Geometry check sheet. Reference: the model listing, model coordinates, mm. Face numbers are marked on the shaded views. A direction names the side the tool comes from. Round coordinates to 2 decimals unless told otherwise and drop trailing zeros. Order: outer loops, then holes, each group sorted by start corner. A loop starts at its lowest first (then second) coordinate and runs counter-clockwise, first axis right, second up. Notation, with made-up numbers: (84.25, -30.5) -> (103.25, -30.5) arc R22 cw to (103.25, -20.5) -> close; hole circle Ø5 at (72.5, 72.25). An arc over 180 degrees is marked (long way). Use a Markdown table: item, result. Add a question column.
Item 1: Material ranges on probe 1 along Z at (x, y) = (0, 3.75); probe 2 along X at (y, z) = (2.25, 0.75); probe 3 along X at (y, z) = (0.5, 1.75), recorded low to high. Write a range as [from, to].
Item 2: Sectioned sample at B-B, the plane z = 0. Record the cut outline in (x, y).
Item 3: Sectioned sample at A-A, the plane x = -11. Record the cut outline in (y, z), and give its area (3 significant figures).
Item 4: Gauge pin test, flat ends, axial feed: pin 1 Ø3 at (y, z) = (8, -1.5) entering from +X; pin 2 Ø0.8 at (x, z) = (0.5, -0.5) entering from +Y. Record the tip position at first contact, or that the pin passes through.
Item 5: Sectioned sample at D-D, the plane y = 4.75. Record the cut outline in (x, z), and give its area (3 significant figures).
Item 6: Sectioned sample at C-C, the plane x = 0. Record the cut outline in (y, z).
Item 7: Set-up check for the marked faces 1 and 2: record each of +Z, -Z, +X, -X, +Y, -Y from which the full face is reachable in a straight line by a thin tool's end or side.
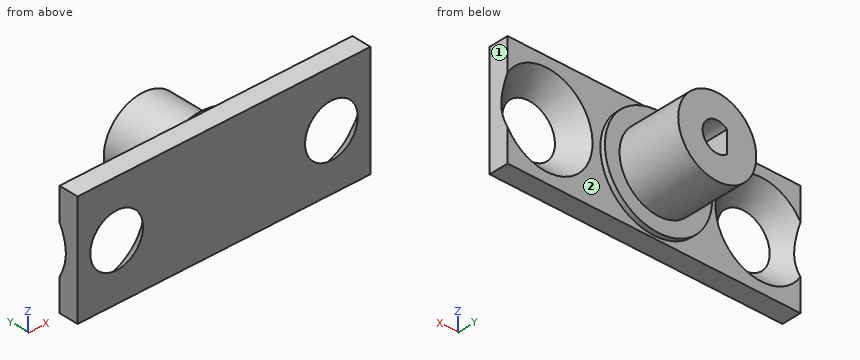
from build123d import *

# Parameters (mm, degrees)
SKETCH1_W                                    = 30
SKETCH1_H                                    = 11.5
BOSS_EXTRUDE1_DEPTH                          = 2
SKETCH2_R                                    = 5.5
BOSS_EXTRUDE2_DEPTH                          = 0.5
SKETCH3_R                                    = 4
BOSS_EXTRUDE3_DEPTH                          = 6.5
CUT_EXTRUDE1_DEPTH                           = 7
CSK_FOR_M4_COUNTERSUNK_FLAT_HEAD_SCR_2_COUNT = 2
CSK_FOR_M4_COUNTERSUNK_FLAT_HEAD_SCR_2_PITCH = 22


with BuildPart() as part:
    # Sketch1 → Boss-Extrude1 (new body)
    with BuildSketch(Plane(origin=(0, 0, 0), x_dir=(1, 0, 0), z_dir=(0, 1, 0))):
        Rectangle(SKETCH1_W, SKETCH1_H)
    extrude(amount=BOSS_EXTRUDE1_DEPTH)

    # Sketch2 → Boss-Extrude2 (add)
    with BuildSketch(Plane(origin=(0, 2, 0), x_dir=(1, 0, 0), z_dir=(0, 1, 0))):
        Circle(SKETCH2_R)
    extrude(amount=BOSS_EXTRUDE2_DEPTH)

    # Sketch3 → Boss-Extrude3 (add)
    with BuildSketch(Plane(origin=(0, 2.5, 0), x_dir=(1, 0, 0), z_dir=(0, 1, 0))):
        Circle(SKETCH3_R)
    extrude(amount=BOSS_EXTRUDE3_DEPTH)

    # Sketch4 → Cut-Extrude1 (cut)
    with BuildSketch(Plane(origin=(0, 9, 0), x_dir=(1, 0, 0), z_dir=(0, 1, 0))):
        with BuildLine():
            Line((-1, 1.118033989), (-1, -1.118033989))
            ThreePointArc((-1, -1.118033989), (1.5, 0), (-1, 1.118033989))
        make_face()
    extrude(amount=-CUT_EXTRUDE1_DEPTH, mode=Mode.SUBTRACT)

    # Sketch6 → CSK for M4 Countersunk Flat Head Screw1 (revolve, cut)
    with BuildSketch(Plane(origin=(11, 2, 0), x_dir=(0, 0, 1), z_dir=(1, 0, 0))):
        Polygon((0, 0), (0, 3.351936393), (2.25, 2), (2.25, 2.45), (4.7, 0), align=None)
    csk_for_m4_countersunk_flat_head_screw1 = revolve(axis=Axis((11, 8.35, 0), (0, -1, 0)), mode=Mode.SUBTRACT)

    # CSK for M4 Countersunk Flat Head Scr 2: CSK for M4 Countersunk Flat Head Screw1 ×2
    with Locations(*[(-i * CSK_FOR_M4_COUNTERSUNK_FLAT_HEAD_SCR_2_PITCH, 0, 0) for i in range(1, CSK_FOR_M4_COUNTERSUNK_FLAT_HEAD_SCR_2_COUNT)]):
        add(csk_for_m4_countersunk_flat_head_screw1, mode=Mode.SUBTRACT)


solid = part.part
Found:
| question | item | result |
|---|---|---|
| 1 | probe 1 | z = [-4, -1.5], [1.5, 4] |
| 1 | probe 2 | x = [-5.45, -1], [1.3, 5.45] |
| 1 | probe 3 | x = [-15, -13.68], [-8.32, 8.32], [13.68, 15] |
| 2 | outline | (-15, 0) -> (-13.7, 0) -> (-15, 1.3) -> close; (-8.3, 0) -> (8.3, 0) -> (6.3, 2) -> (5.5, 2) -> (5.5, 2.5) -> (4, 2.5) -> (4, 9) -> (1.5, 9) -> (1.5, 2) -> (-1, 2) -> (-1, 9) -> (-4, 9) -> (-4, 2.5) -> (-5.5, 2.5) -> (-5.5, 2) -> (-6.3, 2) -> close; (13.7, 0) -> (15, 0) -> (15, 1.3) -> close |
| 3 | outline | (0, -5.75) -> (2, -5.75) -> (2, -4.7) -> (0, -2.7) -> close; (0, 2.7) -> (2, 4.7) -> (2, 5.75) -> (0, 5.75) -> close |
| 3 | area | 8.20 mm2 |
| 4 | pin 1 | stops at x = 4 |
| 4 | pin 2 | stops at y = 2 |
| 5 | outline | circle Ø8 at (0, 0); hole (-1, -1.12) arc R1.5 ccw (long way) to (-1, 1.12) -> close |
| 5 | area | 44.0 mm2 |
| 6 | outline | (0, -5.75) -> (2, -5.75) -> (2, -5.5) -> (2.5, -5.5) -> (2.5, -4) -> (9, -4) -> (9, -1.5) -> (2, -1.5) -> (2, 1.5) -> (9, 1.5) -> (9, 4) -> (2.5, 4) -> (2.5, 5.5) -> (2, 5.5) -> (2, 5.75) -> (0, 5.75) -> close |
| 7 | face 1 | +Z, -Z, +X, +Y, -Y |
| 7 | face 2 | +Y |
